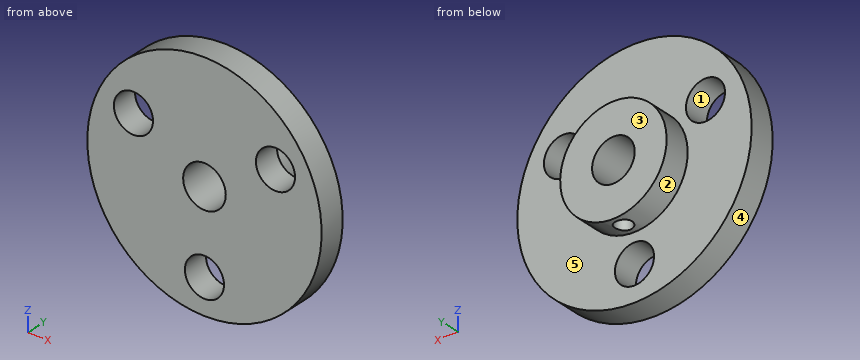
from build123d import *

# Parameters (mm, degrees)
ESBO_O1_R                                      = 11
RESSALTO_EXTRUS_O1_DEPTH                       = 2.5
ESBO_O3_R                                      = 1.835521505
CORTE_EXTRUS_O1_DEPTH                          = 2.5
ESBO_O18_R                                     = 5
RESSALTO_EXTRUS_O5_DEPTH                       = 2.5
ESBO_O20_R                                     = 2
CORTE_EXTRUS_O5_DEPTH                          = 5.5
BROCA_DE_ROSQUEAR_PARA_TARRAXA_DE_M2X0_4_REACH = 21.785
BROCA_DE_ROSQUEAR_PARA_TARRAXA_DE_M2_2_R       = 0.8


with BuildPart() as part:
    # Esboço1 → Ressalto-extrusão1 (new body)
    with BuildSketch(Plane(origin=(0, 0, 0), x_dir=(1, 0, 0), z_dir=(0, 1, 0))):
        with Locations(Location((0, 0, 0), (0, 0, 270))):
            Circle(ESBO_O1_R)
    extrude(amount=RESSALTO_EXTRUS_O1_DEPTH)

    # Esboço3 → Corte-extrusão1 (cut)
    with BuildSketch(Plane(origin=(0, 2.5, 0), x_dir=(1, 0, 0), z_dir=(0, 1, 0))):
        with Locations(Location((0, 7.7, 0), (0, 0, 270))):
            Circle(ESBO_O3_R)
        with Locations(Location((6.668395609, -3.85, 0), (0, 0, 270))):
            Circle(ESBO_O3_R)
        with Locations(Location((-6.668395609, -3.85, 0), (0, 0, 270))):
            Circle(ESBO_O3_R)
    extrude(amount=-CORTE_EXTRUS_O1_DEPTH, mode=Mode.SUBTRACT)

    # Esboço18 → Ressalto-extrusão5 (add)
    with BuildSketch(Plane(origin=(0, 2.5, 0), x_dir=(1, 0, 0), z_dir=(0, 1, 0))):
        with Locations(Location((0, 0, 0), (0, 0, 270))):
            Circle(ESBO_O18_R)
    extrude(amount=RESSALTO_EXTRUS_O5_DEPTH)

    # Esboço20 → Corte-extrusão5 (cut)
    with BuildSketch(Plane(origin=(0, 5, 0), x_dir=(1, 0, 0), z_dir=(0, 1, 0))):
        with Locations(Location((0, 0, 0), (0, 0, 270))):
            Circle(ESBO_O20_R)
    extrude(amount=-CORTE_EXTRUS_O5_DEPTH, mode=Mode.SUBTRACT)

    # Broca de rosquear para tarraxa de M2 2 (on position points) → Broca de rosquear para tarraxa de M2x0.41 (cut, up to next)
    with BuildSketch(Plane(origin=(0.002598781, 3.792959438, -4.999999325), x_dir=(-0.999999864927, 0, -0.000519756122), z_dir=(0.000519756122, 0, -0.999999864927)), mode=Mode.PRIVATE) as broca_de_rosquear_para_tarraxa_de_m2x0_4_sk1:
        Circle(BROCA_DE_ROSQUEAR_PARA_TARRAXA_DE_M2_2_R)
    broca_de_rosquear_para_tarraxa_de_m2x0_4_tool1 = extrude(broca_de_rosquear_para_tarraxa_de_m2x0_4_sk1.sketch, amount=-BROCA_DE_ROSQUEAR_PARA_TARRAXA_DE_M2X0_4_REACH, mode=Mode.PRIVATE) & part.part
    add(broca_de_rosquear_para_tarraxa_de_m2x0_4_tool1.solids().sort_by_distance((0.002599, 3.792959, -4.999999))[0], mode=Mode.SUBTRACT)


solid = part.part
CAD build for the part. Positions are in the model's coordinates, mm. Face numbers are marked on the shaded views. A direction names the side the tool comes from. Round coordinates to 2 decimals unless told otherwise and drop trailing zeros. Order: outer loops, then holes, each group sorted by start corner. A loop starts at its lowest first (then second) coordinate and runs counter-clockwise, first axis right, second up. Notation, with made-up numbers: M 6.5,51.25 L 18.5,51.25 A13 ccw 18.5,67.25 Z; hole C 61,56 d1. An arc over 180 degrees is marked long. Use one line per item in the form item = value.
Q1. Saw through at A-A on z = 0. Give the cut face in (x, y), then the cut area to 3 significant figures.
Recorded:
outline = M -11,0 L -2,0 L -2,5 L -5,5 L -5,2.5 L -11,2.5 Z; M 2,0 L 11,0 L 11,2.5 L 5,2.5 L 5,5 L 2,5 Z
area = 60.0 mm^2
Q2. Saw through at C-C on x = 0. State how many separate pieces and enclosed holes the cut face has, then the cut area to 3 significant figures.
Recorded:
separate_pieces = 4
enclosed_holes = 0
area = 46.0 mm^2
Q3. Saw through at B-B on x = -5.75. Give the cut face in (y, z).
Recorded:
outline = M 0,-9.38 L 2.5,-9.38 L 2.5,2.26 L 0,2.26 Z; M 0,5.44 L 2.5,5.44 L 2.5,9.38 L 0,9.38 Z
Q4. Flat gauge pins, fed straight in: P1, Ø4, axis at x = -6.67, z = 3.85, coming from the +Y side; P2, Ø1.5, axis at y = 4.5, z = -5, coming from the -X side; P3, Ø1.5, axis at y = 3, z = 6, coming from the -X side. Where does each tip first touch, or does it go through?
Recorded:
P1 = 2.5
P2 = -2.63
P3 = -9.56
Q5. Probe L1, parallel to Y at x = -0.25, z = 8.75; L2, parallel to X at y = 1.7, z = -7.7; L3, parallel to Z at x = -5.75, y = 0.85. List the from-to ranges inside material, lowest first.
Recorded:
L1 = 0 to 2.5
L2 = -7.86 to -1.84, 1.84 to 7.86
L3 = -9.38 to 2.26, 5.44 to 9.38
Q6. Two-plate mould, pull along X, no slides. Class the marked faces 1, 2 and 3: +X half, -X half, draft (parallel to the pull), parting line (faces both ways), or undercut.
Recorded:
face_1 = undercut
face_2 = parting line
face_3 = draft
Q7. Which spindle directions (+Z, -Z, +X, -X, +Y, -Y) get a long thin tool onto all of the face, cutting with end or side? Do the marked faces 4 and 5. Say none if no direction does.
Recorded:
face_4 = +Y, -Y
face_5 = +Y
Q8. Saw through at D-D on z = -7.7. Give the cut face in (x, y).
Recorded:
outline = M -7.86,0 L -1.84,0 L -1.84,2.5 L -7.86,2.5 Z; M 1.84,0 L 7.86,0 L 7.86,2.5 L 1.84,2.5 Z
